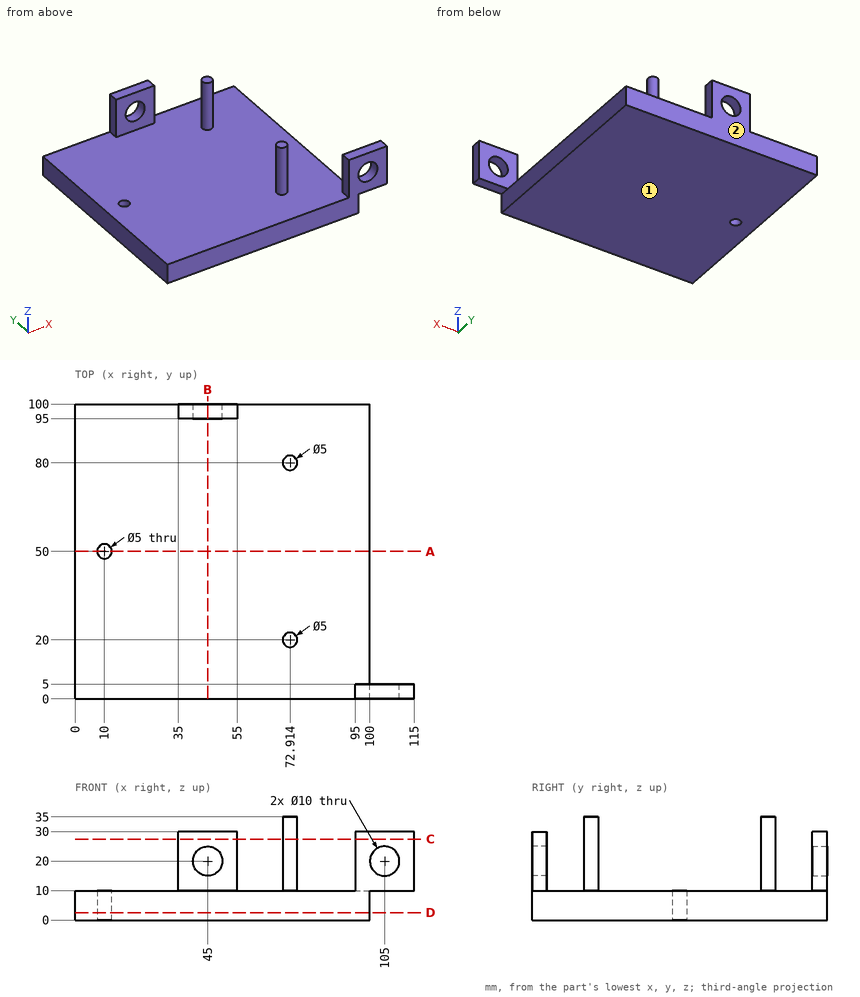
The drawing under review shows one solid part. Ordinate dimensions are in mm from its lowest x, y, z. Round coordinates to 2 decimals unless told otherwise and drop trailing zeros. Loops run counter-clockwise (first coordinate to the right, second up) from the corner with the lowest first, then second, coordinate; pieces in that order, holes last. Notation, with made-up numbers: (-15.5, 14.25) -> (16.5, 14.25) arc R10 cw to (16.5, 30.25) -> close; hole circle Ø10 at (86, -3.5). An arc over 180 degrees is marked (long way). One line per question, with ' | ' between items. Start each with the question number.
Item 1: Draft analysis for pull direction Z (two halves, no side actions). For the marked faces 1 and 2, state which applies: +Z half, -Z half, draft (parallel to the pull), parting line (faces both ways), or undercut.
Item 2: For pin 1 (3 mm diameter, centred on x = 22, y = 77.5, fed in from -Z); pin 2 (10 mm diameter, centred on x = 38.5, z = 26.5, fed in from -Y); pin 3 (8 mm diameter, centred on x = 45, z = 20, fed in from +Y); pin 4 (4 mm diameter, centred on y = 96.5, z = 24, fed in from +X), all flat-tipped, find the tip position at first contact; note any pin that passes through.
Item 3: Wall thickness on line 1 along Z through (x, y) = (45, 97); line 2 along Y through (x, z) = (97, 26); line 3 along Z through (x, y) = (93.5, 4.5): over which ranges is each line inside the solid? List them lowest first. Write a range as [from, to].
Item 4: Add section A-A, the plane y = 50. Write out the cut boundary in (x, z), then the cut area to 3 significant figures.
Item 5: Add section C-C, the plane z = 27.5. Write out the cut boundary in (x, y) (1 decimal), then the cut area to 3 significant figures.
Item 6: Add section B-B, the plane x = 45. Write out the cut boundary in (y, z), then the cut area to 3 significant figures.
Item 7: Add section D-D, the plane z = 2.5. Write out the cut boundary in (x, y), then the cut area to 3 significant figures.
Return value:
1) face 1: -Z half | face 2: draft
2) pin 1: stops at z = 0 | pin 2: stops at y = 95 | pin 3: passes through | pin 4: stops at x = 55
3) line 1: z = [0, 15], [25, 30] | line 2: y = [0, 5] | line 3: z = [0, 10]
4) outline: (0, 0) -> (7.5, 0) -> (7.5, 10) -> (0, 10) -> close; (12.5, 0) -> (100, 0) -> (100, 10) -> (12.5, 10) -> close | area: 950 mm2
5) outline: (35, 95) -> (55, 95) -> (55, 100) -> (35, 100) -> close; circle Ø5 at (72.9, 20); circle Ø5 at (72.9, 80); (95, 0) -> (115, 0) -> (115, 5) -> (95, 5) -> close | area: 239 mm2
6) outline: (0, 0) -> (100, 0) -> (100, 15) -> (95, 15) -> (95, 10) -> (0, 10) -> close; (95, 25) -> (100, 25) -> (100, 30) -> (95, 30) -> close | area: 1,050 mm2
7) outline: (0, 0) -> (100, 0) -> (100, 100) -> (0, 100) -> close; hole circle Ø5 at (10, 50) | area: 9,980 mm2
